from build123d import *

# Parameters (mm, degrees)
F0_W         = 72.464676
F0_H         = 46.138592
F1_DEPTH     = 1.778
F2_R         = 15.875
F4_R         = 13.341257797
F6_R         = 1.1014910557
F7_DEPTH     = 1.27
F9_DEPTH     = 2.032
F10_T1_DEPTH = 15.1513653298
F11_R        = 0.2563999908
F12_DEPTH    = 5.08


# Not quite as in the source:
# - a fillet or chamfer that OpenCascade refuses, or shapes differently, is made with other operations: its cross-section is extruded or revolved along the edge and cut away or added


with BuildPart() as f1:
    # F0 (on Top) → F1 (new body)
    with BuildSketch(Plane.XY):
        Rectangle(F0_W, F0_H)
    extrude(amount=F1_DEPTH)

    # F2 (on face) → F5 section 0
    with BuildSketch(Plane.XY.offset(1.778)):
        Circle(F2_R)
    # F4 (on offset) → F5 section 1
    with BuildSketch(Plane.XY.offset(6.858)):
        Circle(F4_R)
    loft()

    # F6 (on face) → F7 (join)
    with BuildSketch(Plane.XY.offset(6.858)):
        with Locations((7.7888662927, 0)):
            Circle(F6_R)
    extrude(amount=F7_DEPTH)

    # F8 (on face) → F9 (join)
    with BuildSketch(Plane.XY.offset(8.128)):
        with BuildLine():
            Line((6.7317243665, -0.3094082962), (6.7317243665, -5.9662871063))
            Line((6.7317243665, -5.9662871063), (8.8460082188, -5.9662871063))
            Line((8.8460082188, -5.9662871063), (8.8460082188, -0.3094082962))
            ThreePointArc((8.8460082188, -0.3094082962), (7.7888662927, -1.1014910557), (6.7317243665, -0.3094082962))
        make_face()
        with BuildLine():
            Line((6.7317243665, 5.9662871063), (6.7317243665, 0.3094082962))
            ThreePointArc((6.7317243665, 0.3094082962), (7.7888662927, 1.1014910557), (8.8460082188, 0.3094082962))
            Line((8.8460082188, 0.3094082962), (8.8460082188, 5.9662871063))
            Line((8.8460082188, 5.9662871063), (6.7317243665, 5.9662871063))
        make_face()
        with BuildLine():
            Line((6.7317243665, 0.3094082962), (6.7317243665, -0.3094082962))
            ThreePointArc((6.7317243665, -0.3094082962), (7.7888662927, -1.1014910557), (8.8460082188, -0.3094082962))
            Line((8.8460082188, -0.3094082962), (8.8460082188, 0.3094082962))
            ThreePointArc((8.8460082188, 0.3094082962), (7.7888662927, 1.1014910557), (6.7317243665, 0.3094082962))
        make_face()
    extrude(amount=F9_DEPTH)

    # F10: chamfer of 5.08 x 3.5570542941 on 2 edges, made by hand

    # F10_s2 → F10_t1 (cut)
    with BuildSketch(Plane.XY.offset(8.128)):
        Polygon((8.8460082188, -0.8862871063), (5.2889539247, -5.9662871063), (8.8460082188, -5.9662871063), align=None)
        Polygon((8.8460082188, 0.8862871063), (5.2889539247, 5.9662871063), (8.8460082188, 5.9662871063), align=None)
    extrude(amount=F10_T1_DEPTH, mode=Mode.SUBTRACT)

    # F11 (on face) → F12 (join)
    with BuildSketch(Plane.YZ.offset(8.8460082188)):
        with Locations((0, 9.1775208712)):
            Circle(F11_R)
    extrude(amount=F12_DEPTH)


solid = f1.part
Work out the finished part from the listing and answer in its coordinate system (mm). A direction names the side the tool comes from. Round coordinates to 2 decimals unless told otherwise and drop trailing zeros. Loops run counter-clockwise (first coordinate to the right, second up) from the corner with the lowest first, then second, coordinate; pieces in that order, holes last. Notation, with made-up numbers: M -29,-37 L 15,-37 A4 ccw 15,-30 Z; hole C 30.25,75.5 d11. An arc over 180 degrees is marked long. One line per question, with ' | ' between items. Start each with the question number.
(1) A cutting plane is placed at C-C on z = 4.5. Write down the section's boundary in (x, y), plus the area to 3 significant figures.
(2) A cutting plane is placed at B-B on y = 18. Write down the section's boundary in (x, z).
(3) Flat-ended cylindrical pins translate along their axes: pin 1 Ø10 at (x, y) = (-11.5, 2) entering from +Z; pin 2 Ø1.9 at (y, z) = (0, 9) entering from +X; pin 3 Ø1 at (y, z) = (-0.5, 9) entering from -X. Find the tip coordinate at first contact, or state that the pin passes through.
(4) Find the intervals of material crossed by line 1 (Z direction, x = -4, y = -1.5); line 2 (Z direction, x = -5, y = 18); line 3 (X direction, y = -0.5, z = 3.5), in increasing order.
(5) A cutting plane is placed at D-D on x = -20.5. Write down the section's boundary in (y, z), plus the area to 3 significant figures.
(6) For a pull along Z with two mould halves and no side action, classify faces 1 (the face through (-17, 0, 1.778)), 2 (the face through (8.806, -0.422, 7.484)), 3 (the face through (7.804, -2.375, 9.13)) as released by +Z, released by -Z, zero draft, split by the parting line, or undercut.
(7) A cutting plane is placed at A-A on x = 0. Write down the section's boundary in (y, z) (3 decimals).
(8) A tool of negligible diameter and unlimited length cuts with its end or side. For faces 4 (the face through (7.804, 2.375, 9.13)), 5 (the face through (6.732, 0, 9)), 6 (the face through (-1, 0, 0)), from which of +Z, -Z, +X, -X, +Y, -Y can it reach the whole face along a straight path? Write none if from no direction.
Geometry check:
1) outline: C 0,0 d29.03 | area: 662 mm²
2) outline: M -36.23,0 L 36.23,0 L 36.23,1.78 L -36.23,1.78 Z
3) pin 1: stops at z = 6.86 | pin 2: stops at x = 13.93 | pin 3: stops at x = 6.73
4) line 1: z = 0 to 6.86 | line 2: z = 0 to 1.78 | line 3: x = -15.01 to 15.01
5) outline: M -23.07,0 L 23.07,0 L 23.07,1.78 L -23.07,1.78 Z | area: 82.0 mm²
6) face 1: released by +Z | face 2: undercut | face 3: zero draft
7) outline: M -23.069,0 L 23.069,0 L 23.069,1.778 L 15.875,1.778 L 13.341,6.858 L -13.341,6.858 L -15.875,1.778 L -23.069,1.778 Z
8) face 4: +Z, +X, +Y | face 5: +Z, -X, +Y, -Y | face 6: -Z, +X, -X, +Y, -Y
